Could you check a few things on this model? Use its own coordinates, in mm. Coordinates: 2 decimals unless noted, no trailing zeros. Order: outer loops, then holes, each group sorted by start corner. A loop starts at its lowest first (then second) coordinate and runs counter-clockwise, first axis right, second up. Notation, with made-up numbers: M 8,-7.5 L 49,-7.5 A24 ccw 49,29.5 Z; hole C -13.5,86.5 d2. An arc over 180 degrees is marked long. Put each result on its own line as item: value. Start each with the question number.
```python
from build123d import *

# Parameters (mm, degrees)
F1_DEPTH = 152.4
F2_R     = 6.35


with BuildPart() as f1:
    # F0 (on Front) → F1 (new body)
    with BuildSketch(Plane.XZ):
        with BuildLine():
            Line((-133.35, -76.2), (133.35, -76.2))
            Line((133.35, -76.2), (133.35, 0))
            Line((133.35, 0), (82.55, 0))
            ThreePointArc((82.55, 0), (63.5, -19.05), (44.45, 0))
            Line((44.45, 0), (19.05, 0))
            ThreePointArc((19.05, 0), (0, -19.05), (-19.05, 0))
            Line((-19.05, 0), (-44.45, 0))
            ThreePointArc((-44.45, 0), (-63.5, -19.05), (-82.55, 0))
            Line((-82.55, 0), (-133.35, 0))
            Line((-133.35, 0), (-133.35, -76.2))
        make_face()
        with BuildLine():
            Line((82.55, 0), (133.35, 0))
            Line((133.35, 0), (133.35, 76.2))
            Line((133.35, 76.2), (-133.35, 76.2))
            Line((-133.35, 76.2), (-133.35, 0))
            Line((-133.35, 0), (-82.55, 0))
            ThreePointArc((-82.55, 0), (-63.5, 19.05), (-44.45, 0))
            Line((-44.45, 0), (-19.05, 0))
            ThreePointArc((-19.05, 0), (0, 19.05), (19.05, 0))
            Line((19.05, 0), (44.45, 0))
            ThreePointArc((44.45, 0), (63.5, 19.05), (82.55, 0))
        make_face()
    extrude(amount=F1_DEPTH)

    # F2
    f2_edges = [f1.edges().sort_by_distance(p)[0] for p in [
        (0, -152.4, 76.2),
        (133.35, -152.4, 0),
        (-133.35, -152.4, 0),
        (0, -152.4, -76.2),
        (133.35, 0, 0),
        (133.35, -76.2, -76.2),
        (133.35, -76.2, 76.2),
        (-133.35, -76.2, 76.2),
        (0, 0, 76.2),
        (-133.35, -76.2, -76.2),
        (-133.35, 0, 0),
        (0, 0, -76.2),
    ]]
    fillet(f2_edges, radius=F2_R)


solid = f1.part
```
Item 1: If we section it at A-A on z = 0: Write out the boundary of the cut face in (x, y), then the cut area to 3 significant figures.
Item 2: If we section it at C-C on x = 63.5: Write out the boundary of the cut face in (y, z), then the cut area to 3 significant figures.
Item 3: I need wall thicknesses on probe 1 along Z at (x, y) = (0, -95.5); probe 2 along X at (y, z) = (-77.5, -14.5); probe 3 along Z at (x, y) = (66, -23). Which ranges of each line are inside material? Lowest first, please.
Item 4: If we section it at B-B on y = -58.5: Write out the boundary of the cut face in (x, z), then the cut area to 3 significant figures.
Item 5: If we mould it in two halves opening along Z, with no side actions, what happens to faces 1 (the cylindrical face through (131.54, -150.49, 0.98)), 2 (the flat face through (2, -75, 76.2)), 3 (the cylindrical face through (82.53, -75.13, 0.84)), 4 (the cylindrical face through (-44.47, -75.13, 0.84))? For each: released by +Z, released by -Z, zero draft, split by the parting line, or undercut.
Geometry check:
1. outline: M -133.35,-146.05 A6.35 ccw -127,-152.4 L -82.55,-152.4 L -82.55,0 L -127,0 A6.35 ccw -133.35,-6.35 Z; M -44.45,-152.4 L -19.05,-152.4 L -19.05,0 L -44.45,0 Z; M 19.05,-152.4 L 44.45,-152.4 L 44.45,0 L 19.05,0 Z; M 82.55,-152.4 L 127,-152.4 A6.35 ccw 133.35,-146.05 L 133.35,-6.35 A6.35 ccw 127,0 L 82.55,0 Z
1. area: 23,200 mm²
2. outline: M -152.4,-69.85 A6.35 ccw -146.05,-76.2 L -6.35,-76.2 A6.35 ccw 0,-69.85 L 0,-19.05 L -152.4,-19.05 Z; M -152.4,19.05 L 0,19.05 L 0,69.85 A6.35 ccw -6.35,76.2 L -146.05,76.2 A6.35 ccw -152.4,69.85 Z
2. area: 17,400 mm²
3. probe 1: z = -76.2 to -19.05, 19.05 to 76.2
3. probe 2: x = -133.35 to -75.86, -51.14 to -12.36, 12.36 to 51.14, 75.86 to 133.35
3. probe 3: z = -76.2 to -18.89, 18.89 to 76.2
4. outline: M -133.35,-69.85 A6.35 ccw -127,-76.2 L 127,-76.2 A6.35 ccw 133.35,-69.85 L 133.35,69.85 A6.35 ccw 127,76.2 L -127,76.2 A6.35 ccw -133.35,69.85 Z; hole C -63.5,0 d38.1; hole C 0,0 d38.1; hole C 63.5,0 d38.1
4. area: 37,200 mm²
5. face 1: zero draft
5. face 2: released by +Z
5. face 3: undercut
5. face 4: undercut
